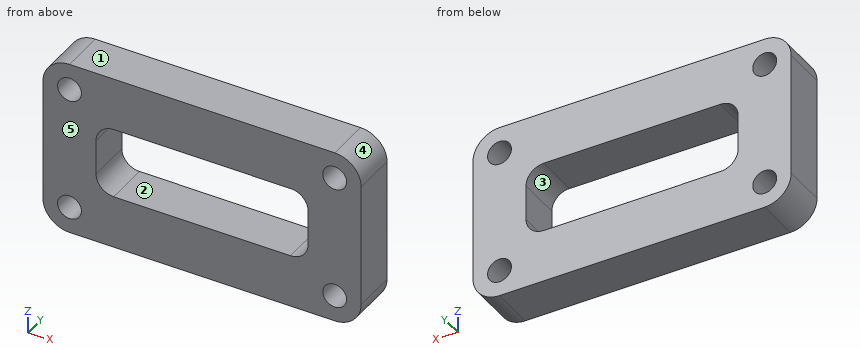
from build123d import *

# Parameters (mm, degrees)
SKETCH_1_W      = 36
SKETCH_1_H      = 20
SKETCH_1_R      = 1.35
SKETCH_1_W_2    = 24
SKETCH_1_H_2    = 8
EXTRUDE_1_DEPTH = 5
FILLET_1_R      = 3
FILLET_2_R      = 2


with BuildPart() as part:
    # 草图1 → 凸台-拉伸1 (new body)
    with BuildSketch(Plane(origin=(0, 0, 0), x_dir=(1, 0, 0), z_dir=(0, 1, 0))):
        with Locations((18, 10)):
            Rectangle(SKETCH_1_W, SKETCH_1_H)
        with Locations(Location((3, 17, 0), (0, 0, 270))):
            Circle(SKETCH_1_R, mode=Mode.SUBTRACT)
        with Locations(Location((33, 17, 0), (0, 0, 90))):
            Circle(SKETCH_1_R, mode=Mode.SUBTRACT)
        with Locations(Location((33, 3, 0), (0, 0, 270))):
            Circle(SKETCH_1_R, mode=Mode.SUBTRACT)
        with Locations(Location((3, 3, 0), (0, 0, 90))):
            Circle(SKETCH_1_R, mode=Mode.SUBTRACT)
        with Locations((18, 10)):
            Rectangle(SKETCH_1_W_2, SKETCH_1_H_2, mode=Mode.SUBTRACT)
    extrude(amount=EXTRUDE_1_DEPTH)

    # 圆角1
    fillet_1_edges = [part.edges().sort_by_distance(p)[0] for p in [
        (0, 2.5, -20),
        (36, 2.5, -20),
        (36, 2.5, 0),
        (0, 2.5, 0),
    ]]
    fillet(fillet_1_edges, radius=FILLET_1_R)

    # 圆角2
    fillet_2_edges = [part.edges().sort_by_distance(p)[0] for p in [
        (6, 2.5, -6),
        (30, 2.5, -6),
        (30, 2.5, -14),
        (6, 2.5, -14),
    ]]
    fillet(fillet_2_edges, radius=FILLET_2_R)


solid = part.part
Here's how the part is built. I have some questions about the finished solid (model axes, mm). Face numbers are marked on the shaded views. A direction names the side the tool comes from. Give positions to 0.01 mm unless a question says otherwise; leave off trailing zeros. Loops run counter-clockwise (first coordinate to the right, second up) from the corner with the lowest first, then second, coordinate; pieces in that order, holes last. Notation, with made-up numbers: (77.25, -21) -> (110.25, -21) arc R14 cw to (110.25, -8) -> close; hole circle Ø2 at (0, -10.5). An arc over 180 degrees is marked (long way). Answer as a JSON object with one key per item and string values. Group by question number.
Item 1: Will this pin go through, and if not, where does the flat tip stop? pin 1 (1.6 mm diameter, centred on x = 3, z = -3, fed in from -Y).
Item 2: On a 3-axis mill with a long thin cutter (end or side, diameter ignored), from which of +Z, -Z, +X, -X, +Y, -Y can I reach the whole of each face in a straight line? I mean the marked faces 1 and 2. Say none if no direction works.
Item 3: Thinking about a two-plate mould opening in X: for the marked faces 3, 4 and 5, which applies, pulls with the +X half, pulls with the -X half, needs draft (parallel to the pull), parting line crosses it, or undercut?
Item 4: Imagine slicing it at A-A on z = -8.5. Write out the boundary of the cut face in (x, y), then the cut area to 3 significant figures.
Item 5: I need wall thicknesses on L1, parallel to X at y = 3, z = -17; L2, parallel to Z at x = 8, y = 1.7; L3, parallel to X at y = 4.05, z = -10.75. Which ranges of each line are inside material? Lowest first, please.
Item 6: Imagine slicing it at C-C on y = 4.25. Write out the boundary of the cut face in (x, z), then the cut area to 3 significant figures.
Item 7: Imagine slicing it at B-B on x = 8.5. Write out the boundary of the cut face in (y, z).
Item 8: Imagine slicing it at D-D on x = 32.5. Write out the boundary of the cut face in (y, z), then the cut area to 3 significant figures.
Answer list:
{
 "1": {"pin 1": "passes through"},
 "2": {"face 1": "+Z, +X, -X, +Y, -Y", "face 2": "+Y, -Y"},
 "3": {"face 3": "undercut", "face 4": "pulls with the +X half", "face 5": "needs draft"},
 "4": {"outline": "(0, 0) -> (6, 0) -> (6, 5) -> (0, 5) -> close; (30, 0) -> (36, 0) -> (36, 5) -> (30, 5) -> close", "area": "60.0 mm2"},
 "5": {"L1": "x = 0 to 1.65, 4.35 to 31.65, 34.35 to 36", "L2": "z = -20 to -14, -6 to 0", "L3": "x = 0 to 6, 30 to 36"},
 "6": {"outline": "(0, -17) arc R3 ccw to (3, -20) -> (33, -20) arc R3 ccw to (36, -17) -> (36, -3) arc R3 ccw to (33, 0) -> (3, 0) arc R3 ccw to (0, -3) -> close; hole circle Ø2.7 at (3, -17); hole circle Ø2.7 at (3, -3); hole (6, -12) arc R2 ccw to (8, -14) -> (28, -14) arc R2 ccw to (30, -12) -> (30, -8) arc R2 ccw to (28, -6) -> (8, -6) arc R2 ccw to (6, -8) -> close; hole circle Ø2.7 at (33, -17); hole circle Ø2.7 at (33, -3)", "area": "501 mm2"},
 "7": {"outline": "(0, -20) -> (5, -20) -> (5, -14) -> (0, -14) -> close; (0, -6) -> (5, -6) -> (5, 0) -> (0, 0) -> close"},
 "8": {"outline": "(0, -20) -> (5, -20) -> (5, -18.25) -> (0, -18.25) -> close; (0, -15.75) -> (5, -15.75) -> (5, -4.25) -> (0, -4.25) -> close; (0, -1.75) -> (5, -1.75) -> (5, 0) -> (0, 0) -> close", "area": "74.9 mm2"}
}
